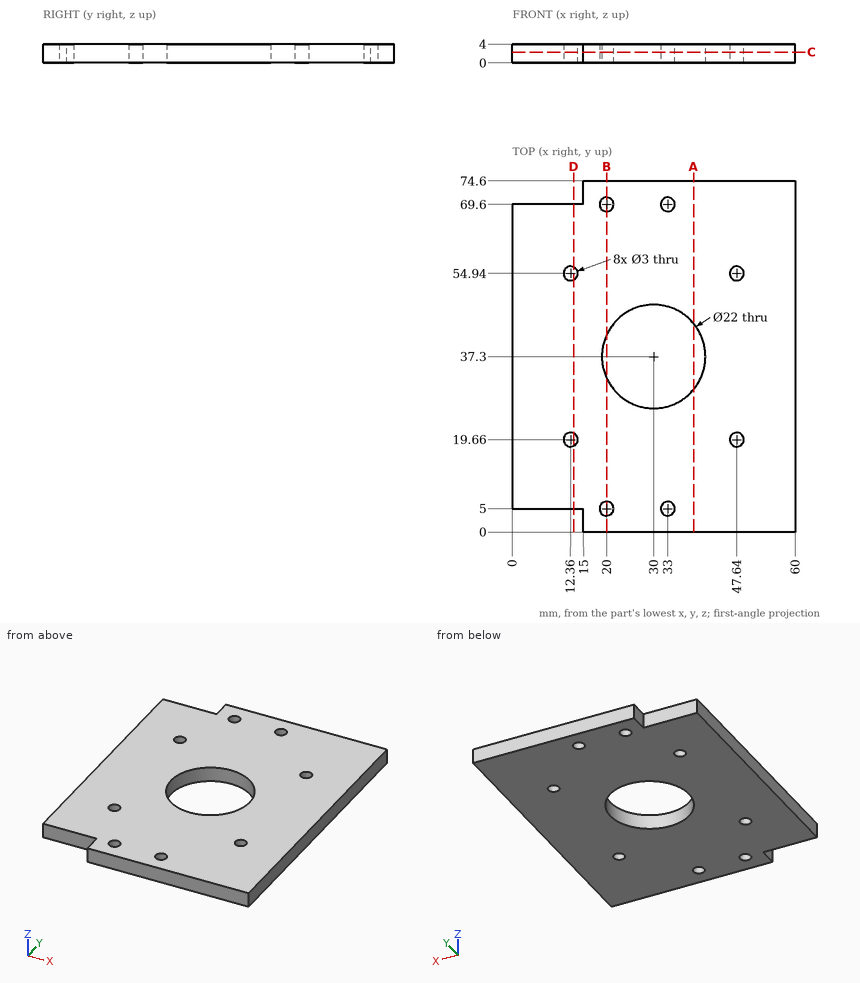
Design review of the part shown in the three views and the two pictorial views. Dimensions are in mm from the part's minimum x, y and z. Coordinates: 2 decimals unless noted, no trailing zeros. Order: outer loops, then holes, each group sorted by start corner. A loop starts at its lowest first (then second) coordinate and runs counter-clockwise, first axis right, second up.
1) Wall thickness on line 1 along Y through (x, z) = (30, 1.5); line 2 along Y through (x, z) = (32, 1.6); line 3 along Y through (x, z) = (20, 2.1): over which ranges is each line inside the solid? List them lowest first.
2) Take a section at B-B, the plane x = 20. Give the boundary of the cut face in (y, z).
3) Take a section at C-C, the plane z = 2.25. State how many separate pieces and enclosed holes the cut face has, and give its area (3 significant figures).
4) Take a section at A-A, the plane x = 38.5. Give the boundary of the cut face in (y, z).
5) Clearance check with flat-ended pins moving along their axes: pin 1 (4 mm diameter, centred on x = 33, y = 69.6, fed in from +Z); pin 2 (2.5 mm diameter, centred on x = 20, y = 69.6, fed in from +Z); pin 3 (2 mm diameter, centred on x = 10, z = 2.5, fed in from -Y); pin 4 (1.2 mm diameter, centred on y = 2.5, z = 1.5, fed in from -X). State where each tip first meets the part, or that it passes through.
6) Take a section at D-D, the plane x = 13. Give the boundary of the cut face in (y, z).
Returned:
1. line 1: y = 0 to 26.3, 48.3 to 74.6
1. line 2: y = 0 to 3.88, 6.12 to 26.48, 48.12 to 68.48, 70.72 to 74.6
1. line 3: y = 0 to 3.5, 6.5 to 32.72, 41.88 to 68.1, 71.1 to 74.6
2. outline: (0, 0) - (3.5, 0) - (3.5, 4) - (0, 4) - close; (6.5, 0) - (32.72, 0) - (32.72, 4) - (6.5, 4) - close; (41.88, 0) - (68.1, 0) - (68.1, 4) - (41.88, 4) - close; (71.1, 0) - (74.6, 0) - (74.6, 4) - (71.1, 4) - close
3. separate pieces: 1
3. enclosed holes: 9
3. area: 3,890 mm2
4. outline: (0, 0) - (30.32, 0) - (30.32, 4) - (0, 4) - close; (44.28, 0) - (74.6, 0) - (74.6, 4) - (44.28, 4) - close
5. pin 1: stops at z = 4
5. pin 2: passes through
5. pin 3: stops at y = 5
5. pin 4: stops at x = 15
6. outline: (5, 0) - (18.3, 0) - (18.3, 4) - (5, 4) - close; (21.02, 0) - (53.58, 0) - (53.58, 4) - (21.02, 4) - close; (56.3, 0) - (69.6, 0) - (69.6, 4) - (56.3, 4) - close
